Can you work these out from the model? Positions are in its coordinate system, mm. Give positions to 0.01 mm unless a question says otherwise; leave off trailing zeros. Loops run counter-clockwise (first coordinate to the right, second up) from the corner with the lowest first, then second, coordinate; pieces in that order, holes last. Notation, with made-up numbers: (-15, 20) - (43, 20) arc R26 ccw to (43, 54) - close; hole circle Ø6 at (51.5, 89). An arc over 180 degrees is marked (long way). Use a Markdown table: item, result. Add a question column.
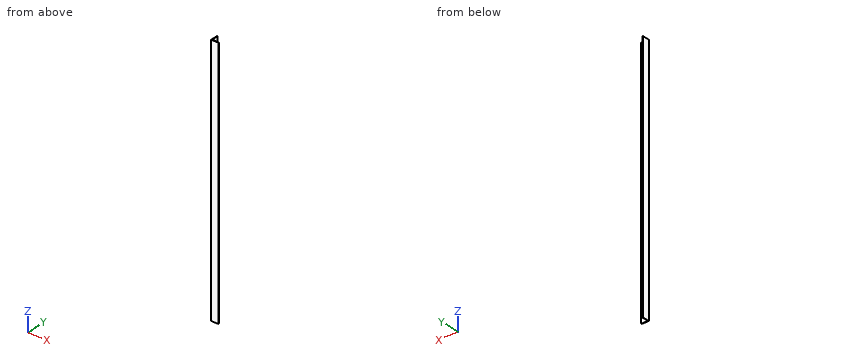
Autodesk Inventor part; units mm, degrees
ref_plane "YZ Plane" through (0, 0, 0) normal (1, 0, 0) x (0, 1, 0)
ref_plane "XZ Plane" through (0, 0, 0) normal (0, 1, 0) x (-1, 0, 0)
ref_plane "XY Plane" through (0, 0, 0) normal (0, 0, 1) x (1, 0, 0)
sketch "Sketch2" plane through (0, 0, 0) normal (0, 0, 1) x (1, 0, 0)
  line L0 (0, 0) -> (1.5, 0)
  line L1 (1.5, 0) -> (1.5, 19)
  line L2 (1.5, 19) -> (0, 19)
  line L3 (0, 19) -> (0, 0)
  line L4 (0, 0) -> (19, 0)
  line L5 (19, 0) -> (19, 1.5)
  line L6 (19, 1.5) -> (0, 1.5)
  line L7 (0, 1.5) -> (0, 0)
  point P0 (1.5, 1.5)
  dimension "d0" = 1.5
  dimension "d1" = 19
  dimension "d2" = 19
  dimension "d3" = 1.5
extrude "Extrusion1" add sketch "Sketch2" along normal mid plane 670
properties part number "GUIA_CANALETA"
1. Will these pins go through, and if not, where does the flat tip stop? P1, Ø1, axis at x = 12.5, z = -21, coming from the +Y side; P2, Ø2, axis at y = 7, z = 251.5, coming from the +X side.
2. Suppose I cut it at B-B (x = 12). List the corners of the cut face in (y, z) for me, and give its area (4 significant figures).
3. Suppose I cut it at A-A (z = 220). List the corners of the cut face in (x, y) for me.
4. Please list where this line runs through material, in increasing order: line 1 along X through (y, z) = (3.5, -296). Write a range as [from, to].
Results below:
| question | item | result |
|---|---|---|
| 1 | P1 | y = 1.5 |
| 1 | P2 | x = 1.5 |
| 2 | outline | (0, -335) - (1.5, -335) - (1.5, 335) - (0, 335) - close |
| 2 | area | 1,005 mm² |
| 3 | outline | (0, 0) - (19, 0) - (19, 1.5) - (1.5, 1.5) - (1.5, 19) - (0, 19) - close |
| 4 | line 1 | [0, 1.5] |
